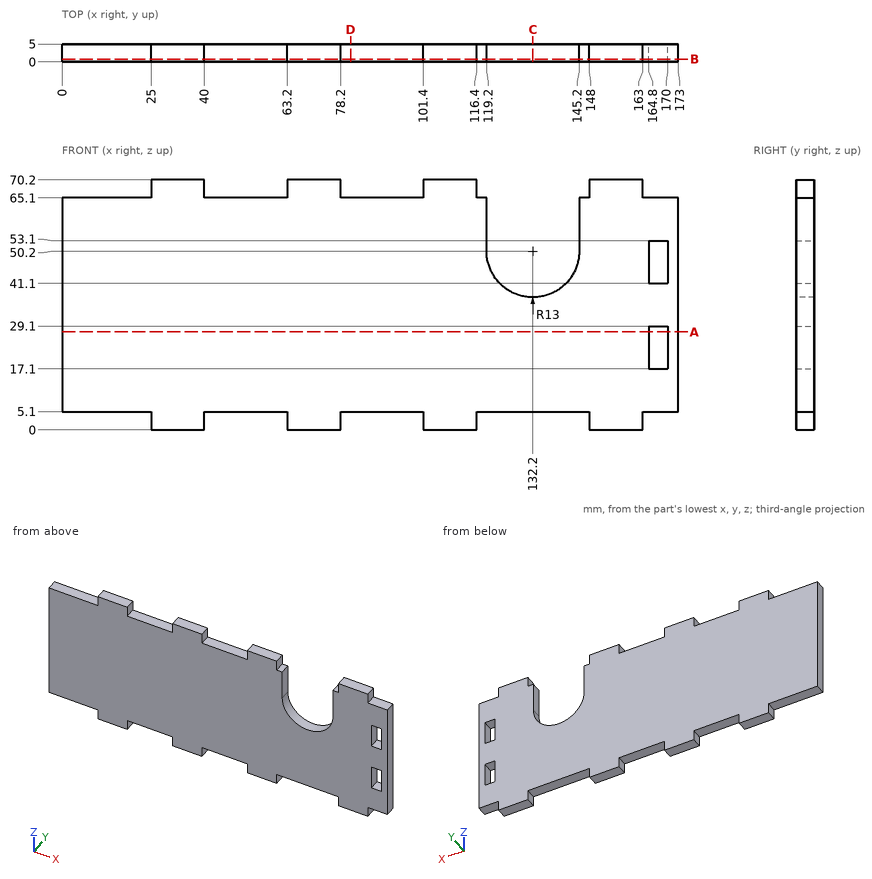
Source: three-view drawing plus pictorial views. Frame: mm from the lowest corner of the part. Round coordinates to 2 decimals unless told otherwise and drop trailing zeros. Loops run counter-clockwise (first coordinate to the right, second up) from the corner with the lowest first, then second, coordinate; pieces in that order, holes last.
Q1. Section C-C on x = 132.2. Return loops of the section in (y, z), plus the area to 4 significant figures.
Q2. Pin query (flat end, axial travel): P1, Ø1.5, axis at x = 169, y = 3, coming from the -Z side; P2, Ø1.5, axis at x = 122, y = 2, coming from the +Z side; P3, Ø2.5, axis at y = 3, z = 2, coming from the +X side. Return the tip coordinate at first contact, or that it passes through.
Q3. Section B-B on y = 0.75. State how many separate pieces and enclosed holes the cut face has, plus the area to 3 significant figures.
Q4. Material intervals for L1, parallel to X at y = 4.25, z = 25; L2, parallel to X at y = 0.3, z = 65.5; L3, parallel to Z at x = 145.5, y = 3.7, sorted ascending.
Q5. Section A-A on z = 27.5. Return loops of the section in (x, y), plus the area to 3 significant figures.
Q6. Section D-D on x = 81. Return loops of the section in (y, z).
Evaluation:
1. outline: (0, 5.1) - (5, 5.1) - (5, 37.2) - (0, 37.2) - close
1. area: 160.5 mm2
2. P1: stops at z = 5.1
2. P2: stops at z = 43.19
2. P3: stops at x = 163
3. separate pieces: 1
3. enclosed holes: 2
3. area: 10,200 mm2
4. L1: x = 0 to 164.8, 170 to 173
4. L2: x = 25 to 40, 63.2 to 78.2, 101.4 to 116.4, 148 to 163
4. L3: z = 5.1 to 65.1
5. outline: (0, 0) - (164.8, 0) - (164.8, 5) - (0, 5) - close; (170, 0) - (173, 0) - (173, 5) - (170, 5) - close
5. area: 839 mm2
6. outline: (0, 5.1) - (5, 5.1) - (5, 65.1) - (0, 65.1) - close
